```python
from build123d import *

# Parameters (mm, degrees)
SKETCH1_R           = 57.5
SKETCH1_R_2         = 1.5
SKETCH1_R_3         = 29
BOSS_EXTRUDE1_DEPTH = 15
BOSS_EXTRUDE2_DEPTH = 115
CUT_EXTRUDE1_START  = -48.6
SKETCH3_R           = 57.5
CUT_EXTRUDE1_DEPTH  = 48.6
SKETCH5_R           = 2
CUT_EXTRUDE3_DEPTH  = 75.6
SKETCH6_R           = 4.25
CUT_EXTRUDE4_DEPTH  = 62.5
CUT_EXTRUDE2_DEPTH  = 132.6
FILLET1_R           = 10


with BuildPart() as part:
    # Sketch1 → Boss-Extrude1 (new body)
    # profile 1 of 3: a face of its own
    with BuildSketch(Plane(origin=(0, 0, 0), x_dir=(1, 0, 0), z_dir=(0, 1, 0))):
        Circle(SKETCH1_R)
        with Locations(Location((-30.000792583, 44.899359064, 0), (0, 0, 270))):
            Circle(SKETCH1_R_2, mode=Mode.SUBTRACT)
        with Locations(Location((-44.899359064, 30.000792583, 0), (0, 0, 270))):
            Circle(SKETCH1_R_2, mode=Mode.SUBTRACT)
        with Locations(Location((-52.962405142, 10.534877389, 0), (0, 0, 270))):
            Circle(SKETCH1_R_2, mode=Mode.SUBTRACT)
        with Locations(Location((-52.962405142, -10.534877389, 0), (0, 0, 270))):
            Circle(SKETCH1_R_2, mode=Mode.SUBTRACT)
        with Locations(Location((-44.899359064, -30.000792583, 0), (0, 0, 270))):
            Circle(SKETCH1_R_2, mode=Mode.SUBTRACT)
        with Locations(Location((-30.000792583, -44.899359064, 0), (0, 0, 270))):
            Circle(SKETCH1_R_2, mode=Mode.SUBTRACT)
        with Locations(Location((-10.534877389, -52.962405142, 0), (0, 0, 270))):
            Circle(SKETCH1_R_2, mode=Mode.SUBTRACT)
        with Locations(Location((10.534877389, -52.962405142, 0), (0, 0, 270))):
            Circle(SKETCH1_R_2, mode=Mode.SUBTRACT)
        with Locations(Location((30.000792583, -44.899359064, 0), (0, 0, 270))):
            Circle(SKETCH1_R_2, mode=Mode.SUBTRACT)
        with Locations(Location((44.899359064, -30.000792583, 0), (0, 0, 270))):
            Circle(SKETCH1_R_2, mode=Mode.SUBTRACT)
        with Locations(Location((52.962405142, -10.534877389, 0), (0, 0, 270))):
            Circle(SKETCH1_R_2, mode=Mode.SUBTRACT)
        with Locations(Location((52.962405142, 10.534877389, 0), (0, 0, 270))):
            Circle(SKETCH1_R_2, mode=Mode.SUBTRACT)
        with Locations(Location((44.899359064, 30.000792583, 0), (0, 0, 270))):
            Circle(SKETCH1_R_2, mode=Mode.SUBTRACT)
        with Locations(Location((30.000792583, 44.899359064, 0), (0, 0, 270))):
            Circle(SKETCH1_R_2, mode=Mode.SUBTRACT)
        with Locations(Location((10.534877389, 52.962405142, 0), (0, 0, 270))):
            Circle(SKETCH1_R_2, mode=Mode.SUBTRACT)
        with Locations(Location((-10.534877389, 52.962405142, 0), (0, 0, 270))):
            Circle(SKETCH1_R_2, mode=Mode.SUBTRACT)
        with Locations(Location((0, 0, 0), (0, 0, 270))):
            Circle(SKETCH1_R_3, mode=Mode.SUBTRACT)
    # profile 2 of 3: a face of its own
    with BuildSketch(Plane(origin=(0, 0, 0), x_dir=(1, 0, 0), z_dir=(0, 1, 0))):
        with BuildLine():
            ThreePointArc((2.7e-08, -57.5), (-40.658639909, -40.658639928), (-57.5, 0))
            Line((-57.5, 0), (-57.5, -57.5))
            Line((-57.5, -57.5), (2.7e-08, -57.5))
        make_face()
    # profile 3 of 3: a face of its own
    with BuildSketch(Plane(origin=(0, 0, 0), x_dir=(1, 0, 0), z_dir=(0, 1, 0))):
        with BuildLine():
            Line((57.5, -57.5), (57.5, 0))
            ThreePointArc((57.5, 0), (40.658639928, -40.658639909), (2.7e-08, -57.5))
            Line((2.7e-08, -57.5), (57.5, -57.5))
        make_face()
    extrude(amount=BOSS_EXTRUDE1_DEPTH)

    # Sketch2 → Boss-Extrude2 (add)
    with BuildSketch(Plane.ZY.offset(57.5)):
        Polygon((57.5, 15), (57.5, 0), (72.5, 0), (72.5, 63.6), (57.5, 63.6), align=None)
        Polygon((0, 15), (57.5, 15), (57.5, 63.6), align=None)
    extrude(amount=-BOSS_EXTRUDE2_DEPTH)

    # Sketch3 → Cut-Extrude1 (cut)
    with BuildSketch(Plane(origin=(0, 63.6, 0), x_dir=(1, 0, 0), z_dir=(0, 1, 0)).offset(CUT_EXTRUDE1_START)):
        Circle(SKETCH3_R)
    extrude(amount=CUT_EXTRUDE1_DEPTH, mode=Mode.SUBTRACT)

    # Sketch5 → Cut-Extrude3 (cut)
    with BuildSketch(Plane.XY.offset(72.5)):
        with Locations((0, 56.6)):
            Circle(SKETCH5_R)
        with Locations((-19.918584287, 45.1)):
            Circle(SKETCH5_R)
        with Locations((-19.918584287, 22.1)):
            Circle(SKETCH5_R)
        with Locations((19.918584287, 22.1)):
            Circle(SKETCH5_R)
        with Locations((19.918584287, 45.1)):
            Circle(SKETCH5_R)
    extrude(amount=-CUT_EXTRUDE3_DEPTH, mode=Mode.SUBTRACT)

    # Sketch6 → Cut-Extrude4 (cut)
    with BuildSketch(Plane.XY):
        with Locations(Location((0, 56.6, 0), (0, 0, 270))):
            Circle(SKETCH6_R)
        with Locations(Location((19.918584287, 45.1, 0), (0, 0, 180))):
            Circle(SKETCH6_R)
        with Locations(Location((19.918584287, 22.1, 0), (0, 0, 180))):
            Circle(SKETCH6_R)
        with Locations(Location((-19.918584287, 22.1, 0), (0, 0, 180))):
            Circle(SKETCH6_R)
        with Locations(Location((-19.918584287, 45.1, 0), (0, 0, 180))):
            Circle(SKETCH6_R)
    extrude(amount=CUT_EXTRUDE4_DEPTH, mode=Mode.SUBTRACT)

    # Sketch4 → Cut-Extrude2 (cut)
    with BuildSketch(Plane.XY.offset(72.5)):
        with BuildLine():
            Line((-57.5, 63.6), (-57.5, 6.099999962))
            ThreePointArc((-57.5, 6.099999962), (-40.658639932, 46.758639905), (0, 63.6))
            Line((0, 63.6), (-57.5, 63.6))
        make_face()
        with BuildLine():
            Line((57.5, 63.6), (0, 63.6))
            ThreePointArc((0, 63.6), (40.658639918, 46.758639918), (57.5, 6.1))
            Line((57.5, 6.1), (57.5, 63.6))
        make_face()
    extrude(amount=-CUT_EXTRUDE2_DEPTH, mode=Mode.SUBTRACT)

    # Fillet1
    fillet1_edges = [part.edges().sort_by_distance(p)[0] for p in [
        (0, 0, 72.5),
    ]]
    fillet(fillet1_edges, radius=FILLET1_R)


solid = part.part
```
Model file for the job. Use its own axes, mm. A direction names the side the tool comes from. Coordinates: 2 decimals unless noted, no trailing zeros. Loops run counter-clockwise (first coordinate to the right, second up) from the corner with the lowest first, then second, coordinate; pieces in that order, holes last. Notation, with made-up numbers: (-31.75, -13) - (22.25, -13) arc R20 ccw to (22.25, -5) - close; hole circle Ø5 at (46.5, 78.5). An arc over 180 degrees is marked (long way). Answer as a JSON object with one key per item and string values. Group by question number.
(1) Cut at A-A (z = 61). Give the cut face in (x, y), then the cut area to 3 significant figures.
(2) Tool access for faces 4 (the face through (10.6, 7.4, -54.46)), 5 (the face through (-26, 15, -14)), 6 (the face through (24.164, 44.913, 58.412)): list every direction of +Z, -Z, +X, -X, +Y, -Y with a clear straight run to the whole face (end or side of a thin tool).
(3) Two-plate mould, pull along X, no slides. Class faces 1 (the face through (1.264, 7.395, -57.486)), 2 (the face through (-51.698, 7.395, 11.341)), 3 (the face through (12, 0, 28)): released by +X, released by -X, zero draft, split by the parting line, or undercut.
(4) Cut at C-C (y = 45.1). Give the cut face in (x, z).
(5) Flat gauge pins, fed straight in: pin 1 (2.5 mm diameter, centred on x = -21.5, y = 21, fed in from -Z); pin 2 (12 mm diameter, centred on x = -44.5, z = 0, fed in from -Y); pin 3 (1.5 mm diameter, centred on x = 23, y = 40.5, fed in from -Z); pin 4 (6 mm diameter, centred on y = 17, z = 28, fed in from +X). Where does each tip first touch, or does it go through?
(6) Probe line 1 along Z through (x, y) = (-44.5, 4); line 2 along Y through (x, z) = (-5, 29.5); line 3 along X through (y, z) = (22, 51). List the from-to ranges inside material, lowest first.
(7) Cut at B-B (x = 6.5). Give the cut face in (y, z), then the cut area to 3 significant figures.
(8) Cut at D-D (y = 56.6). Give the cut face in (x, z).
Geometry says:
{
 "1": {"outline": "(-57.5, 0) - (57.5, 0) - (57.5, 6.1) arc R57.5 ccw to (-57.5, 6.1) - close; hole circle Ø8.5 at (-19.92, 22.1); hole circle Ø8.5 at (-19.92, 45.1); hole circle Ø8.5 at (0, 56.6); hole circle Ø8.5 at (19.92, 22.1); hole circle Ø8.5 at (19.92, 45.1)", "area": "5,610 mm^2"},
 "2": {"face 4": "+Y, -Y", "face 5": "-Z, +Y", "face 6": "-Z"},
 "3": {"face 1": "split by the parting line", "face 2": "undercut", "face 3": "zero draft"},
 "4": {"outline": "(-42.25, 39) arc R57.5 cw to (-24.17, 52.17) - (-24.17, 62.5) - (-21.92, 62.5) - (-21.92, 72.5) - (-42.25, 72.5) - close; (-17.92, 62.5) - (-15.67, 62.5) - (-15.67, 55.32) arc R57.5 cw to (15.67, 55.32) - (15.67, 62.5) - (17.92, 62.5) - (17.92, 72.5) - (-17.92, 72.5) - close; (21.92, 62.5) - (24.17, 62.5) - (24.17, 52.17) arc R57.5 cw to (42.25, 39) - (42.25, 72.5) - (21.92, 72.5) - close"},
 "5": {"pin 1": "stops at z = 62.5", "pin 2": "stops at y = 0", "pin 3": "stops at z = 52.37", "pin 4": "stops at x = 56.95"},
 "6": {"line 1": "z = -36.41 to -31.45, -28.55 to 28.55, 31.45 to 70.5", "line 2": "y = 0 to 15", "line 3": "x = -55.26 to -26.56, 26.56 to 55.26"},
 "7": {"outline": "(0, -57.13) - (15, -57.13) - (15, -28.26) - (0, -28.26) - close; (0, 28.26) - (15, 28.26) - (15, 57.13) - (63.23, 57.13) - (63.23, 72.5) - (10, 72.5) arc R10 ccw to (0, 62.5) - close", "area": "1,820 mm^2"},
 "8": {"outline": "(-27.5, 50.5) arc R57.5 cw to (-4.25, 57.34) - (-4.25, 62.5) - (-2, 62.5) - (-2, 72.5) - (-27.5, 72.5) - close; (2, 62.5) - (4.25, 62.5) - (4.25, 57.34) arc R57.5 cw to (27.5, 50.5) - (27.5, 72.5) - (2, 72.5) - close"}
}
